```python
from build123d import *

# Parameters (mm, degrees)
BOSS_EXTRUDE1_DEPTH = 20
SKETCH2_R           = 21
CUT_EXTRUDE1_DEPTH  = 15
SKETCH3_R           = 3
CUT_EXTRUDE2_DEPTH  = 8
SKETCH4_R           = 3
CUT_EXTRUDE3_DEPTH  = 15
SKETCH5_R           = 3
CUT_EXTRUDE4_DEPTH  = 20
FILLET1_R           = 5
SKETCH6_R           = 3
CUT_EXTRUDE7_DEPTH  = 10


with BuildPart() as part:
    # Sketch1 → Boss-Extrude1 (new body)
    with BuildSketch(Plane.XY):
        Polygon((-200.6, -50), (200.6, -50), (200.6, 50), (60, 50), (60, 250), (-60, 250), (-60, 50), (-200.6, 50), align=None)
    extrude(amount=BOSS_EXTRUDE1_DEPTH)

    # Sketch2 → Cut-Extrude1 (cut)
    with BuildSketch(Plane.XY.offset(20)):
        with Locations((167.7, 0)):
            Circle(SKETCH2_R)
        with Locations(Location((-167.7, 0, 0), (0, 0, 180))):
            Circle(SKETCH2_R)
    extrude(amount=-CUT_EXTRUDE1_DEPTH, mode=Mode.SUBTRACT)

    # Sketch3 → Cut-Extrude2 (cut)
    with BuildSketch(Plane.XY.offset(20)):
        with Locations((-35, 97.753157488)):
            Circle(SKETCH3_R)
        with Locations((35, 97.753157488)):
            Circle(SKETCH3_R)
        with Locations((0, 97.753157488)):
            Circle(SKETCH3_R)
    extrude(amount=-CUT_EXTRUDE2_DEPTH, mode=Mode.SUBTRACT)

    # Sketch4 → Cut-Extrude3 (cut)
    with BuildSketch(Plane.XY.offset(20)):
        with Locations((-86, -20.5)):
            Circle(SKETCH4_R)
        with Locations((88.5, -20.5)):
            Circle(SKETCH4_R)
        with Locations((88.5, -34.5)):
            Circle(SKETCH4_R)
        with Locations((-86, -34.5)):
            Circle(SKETCH4_R)
    extrude(amount=-CUT_EXTRUDE3_DEPTH, mode=Mode.SUBTRACT)

    # Sketch5 → Cut-Extrude4 (cut)
    with BuildSketch(Plane.XY.offset(20)):
        with Locations((157.08787293, -42)):
            Circle(SKETCH5_R)
    cut_extrude4 = extrude(amount=-CUT_EXTRUDE4_DEPTH, mode=Mode.SUBTRACT)

    # Mirror2: Cut-Extrude4 across plane
    add(cut_extrude4.mirror(Plane(origin=(0, 0, 0), x_dir=(0, 0, 1), z_dir=(1, 0, 0))), mode=Mode.SUBTRACT)

    # Fillet1
    fillet1_edges = [part.edges().sort_by_distance(p)[0] for p in [
        (-60, 150, 0),
        (0, 250, 0),
        (60, 150, 0),
        (130.3, 50, 0),
        (0, 250, 20),
        (200.6, 50, 10),
        (200.6, -50, 10),
        (-200.6, 50, 10),
        (-60, 250, 10),
        (60, 250, 10),
        (-60, 150, 20),
        (-130.3, 50, 20),
        (-200.6, 0, 20),
        (0, -50, 20),
        (200.6, 0, 20),
        (130.3, 50, 20),
        (200.6, 0, 0),
        (60, 150, 20),
        (0, -50, 0),
        (-130.3, 50, 0),
    ]]
    fillet(fillet1_edges, radius=FILLET1_R - 0.0001)  # a hair under: the kernel refuses the full size

    # Sketch6 → Cut-Extrude7 (cut)
    with BuildSketch(Plane.ZY.offset(60)):
        with Locations(Location((9.525, 210, 0), (0, 0, 270))):
            Circle(SKETCH6_R)
    cut_extrude7 = extrude(amount=-CUT_EXTRUDE7_DEPTH, mode=Mode.SUBTRACT)

    # Mirror3: Cut-Extrude7 across plane
    add(cut_extrude7.mirror(Plane(origin=(0, 0, 0), x_dir=(0, 0, 1), z_dir=(1, 0, 0))), mode=Mode.SUBTRACT)


solid = part.part
```
Here's how the part is built. I have some questions about the finished solid (model axes, mm). A direction names the side the tool comes from. Coordinates: 2 decimals unless noted, no trailing zeros. Write each loop counter-clockwise with the first axis right and the second up, starting at its lowest first coordinate (ties: lowest second). Pieces come first, ordered by that corner, then holes. Notation, with made-up numbers: (-7.5, -11) -> (5.5, -11) arc R34 cw to (5.5, 28) -> close; hole circle Ø10 at (-28.75, 5.25). An arc over 180 degrees is marked (long way). Use a Markdown table: item, result. Add a question column.
(1) If we section it at B-B, the plane y = 0: Write out the boundary of the cut face in (x, z), and give its area (3 significant figures).
(2) If we section it at A-A, the plane x = -95: Write out the boundary of the cut face in (y, z), and give its area (3 significant figures).
(3) I'm going to push flat-ended pins straight in: P1, Ø5, axis at x = 35, y = 97.75, coming from the +Z side; P2, Ø3, axis at y = 210.5, z = 9, coming from the -X side; P3, Ø10, axis at y = 142, z = 18, coming from the -X side; P4, Ø8, axis at x = -147, y = 46.5, coming from the -Z side. Where does each tip first touch, or does it pass through?
(4) For faces 5 (the flat face through (60, 146, 10)), 6 (the flat face through (-60, 149, 10)), 7 (the cylindrical face through (-187.1, 8.04, 12.6)), which set-ups out of +Z, -Z, +X, -X, +Y, -Y let a thin tool reach every point of the face, with its end or its side?
(5) We'd pull the mould along Y, two halves only. Please class faces 1 (the flat face through (-5, -50, 10)), 2 (the flat face through (-127, 50, 10)), 3 (the cylindrical face through (187.1, -8.04, 12.6)), 4 (the flat face through (-200.6, -2, 7)): +Y half, -Y half, draft (parallel to the pull), parting line (faces both ways), or undercut.
(6) Please list where these lines run through material, in increasing order: line 1 (Y direction, x = 35, z = 15.75); line 2 (X direction, y = 1.5, z = 4.75); line 3 (Y direction, x = 122, z = 13.75).
(7) If we section it at C-C, the plane y = 157: Write out the boundary of the cut face in (x, z).
Outcome:
| question | item | result |
|---|---|---|
| 1 | outline | (-200.6, 0) -> (195.6, 0) arc R5 ccw to (200.6, 5) -> (200.6, 15) arc R5 ccw to (195.6, 20) -> (188.7, 20) -> (188.7, 5) -> (146.7, 5) -> (146.7, 20) -> (-146.7, 20) -> (-146.7, 5) -> (-188.7, 5) -> (-188.7, 20) -> (-195.6, 20) arc R5 ccw to (-200.6, 15) -> close |
| 1 | area | 6,750 mm^2 |
| 2 | outline | (-50, 5) arc R5 ccw to (-45, 0) -> (45, 0) arc R5 ccw to (50, 5) -> (50, 15) arc R5 ccw to (45, 20) -> (-45, 20) arc R5 ccw to (-50, 15) -> close |
| 2 | area | 1,980 mm^2 |
| 3 | P1 | stops at z = 12 |
| 3 | P2 | stops at x = -50 |
| 3 | P3 | stops at x = -60 |
| 3 | P4 | stops at z = 0 |
| 4 | face 5 | +Z, -Z, +X, +Y |
| 4 | face 6 | +Z, -Z, -X, +Y |
| 4 | face 7 | +Z |
| 5 | face 1 | -Y half |
| 5 | face 2 | +Y half |
| 5 | face 3 | undercut |
| 5 | face 4 | draft |
| 6 | line 1 | y = -49.94 to 94.75, 100.75 to 249.94 |
| 6 | line 2 | x = -200.6 to 200.59 |
| 6 | line 3 | y = -50 to 50 |
| 7 | outline | (-60, 5) arc R5 ccw to (-55, 0) -> (55, 0) arc R5 ccw to (60, 5) -> (60, 15) arc R5 ccw to (55, 20) -> (-55, 20) arc R5 ccw to (-60, 15) -> close |
